Autodesk Inventor part; units mm, degrees
ref_plane "YZ Plane" through (0, 0, 0) normal (1, 0, 0) x (0, 1, 0)
ref_plane "XZ Plane" through (0, 0, 0) normal (0, 1, 0) x (-1, 0, 0)
ref_plane "XY Plane" through (0, 0, 0) normal (0, 0, 1) x (1, 0, 0)
sketch "Sketch1" plane through (0, 0, 0) normal (0, 0, 1) x (1, 0, 0)
  line L0 (0, 0) -> (419.7625, 0)
  line L1 (419.7625, 0) -> (419.7625, 420)
  line L2 (419.7625, 420) -> (0, 420)
  line L3 (0, 420) -> (0, 0)
  dimension "d0" = 419.7625
  dimension "d1" = 420
extrude "Extrusion1" add sketch "Sketch1" along normal blind 4.7625
sketch "Sketch3" plane through (0, 0, 4.7625) normal (0, 0, 1) x (1, 0, 0)
  line L0 (0, 0) -> (419.7625, 0)
  line L1 (0, 420) -> (0, 0)
  circle A0 centre (209.8815, 40) radius 19.05
  dimension "d13" = 38.1
  dimension "d14" = 209.8815
  dimension "d30" = 40
extrude "Extrusion2" cut sketch "Sketch3" against normal up to next
sketch "Sketch5" plane through (0, 0, 4.7625) normal (0, 0, 1) x (1, 0, 0)
  circle A0 centre (209.8815, 40) radius 19.05
  point P0 (193.8815, 56)
  point P1 (225.8815, 56)
  point P2 (193.8815, 24)
  point P3 (225.8815, 24)
  dimension "d31" = 32
  dimension "d32" = 32
  dimension "d33" = 16
  dimension "d34" = 16
hole "Hole2" at (193.8815, 56, 4.7625) at (225.8815, 56, 4.7625) at (193.8815, 24, 4.7625) at (225.8815, 24, 4.7625) direction (0, 0, -1) diameter 3.5 end through all
sketch "Sketch6" plane through (0, 0, 4.7625) normal (0, 0, 1) x (1, 0, 0)
  line L0 (0, 0) -> (419.7625, 0)
  line L1 (419.7625, 0) -> (419.7625, 420)
  line L2 (419.7625, 420) -> (0, 420)
  line L3 (0, 420) -> (0, 0)
  circle A0 centre (10, 410) radius 2.25
  circle A1 centre (409.7625, 410) radius 2.25
  circle A2 centre (10, 10) radius 2.25
  circle A3 centre (409.7625, 10) radius 2.25
  circle A4 centre (10, 210) radius 2.25
  circle A5 centre (409.7625, 210) radius 2.25
  circle A6 centre (209.8815, 410) radius 2.25
  circle A7 centre (209.8815, 10) radius 2.25
  circle A8 centre (209.8815, 75) radius 2.25
  dimension "d42" = 4.5
  dimension "d43" = 10
  dimension "d44" = 10
  dimension "d45" = 10
  dimension "d46" = 10
  dimension "d47" = 10
  dimension "d48" = 210
  dimension "d51" = 209.8815
  dimension "d55" = 75
extrude "Extrusion3" cut sketch "Sketch6" against normal up to next contours A0 | A1 | A2 | A3 | A4 | A5 | A6 | A7 | A8
chamfer "Chamfer1" distance 2 angle 45 9 edges at (7.75, 410, 4.7625) (207.6315, 410, 4.7625) (407.5125, 410, 4.7625) (407.5125, 210, 4.7625) (7.75, 210, 4.7625) (7.75, 10, 4.7625) (207.6315, 10, 4.7625) (407.5125, 10, 4.7625) (207.6315, 75, 4.7625)
properties part number "EnclosurePanelSide" material "ABS Plastic"
Work out the finished part from the listing and answer in its coordinate system (mm). Coordinates: 2 decimals unless noted, no trailing zeros. Use a Markdown table: item, result.
Item 1: Given pin 1 Ø2 at (x, y) = (225.88, 24) entering from +Z; pin 2 Ø6 at (x, y) = (409.76, 10) entering from +Z (3 decimals); pin 3 Ø5 at (x, y) = (10, 410) entering from +Z; pin 4 Ø7 at (x, y) = (10, 10) entering from +Z, each flat-ended and moving along its own axis, determine where each tip first touches the part or whether it passes through.
Evaluation:
| item | result |
|---|---|
| pin 1 | passes through |
| pin 2 | stops at z = 3.515 |
| pin 3 | stops at z = 3.01 |
| pin 4 | stops at z = 4.01 |
Item 2: The mould has two halves that part along Y. Classify faces 1 (the flat face through (207, 213, 0)), 2 (the cylindrical face through (228.052, 45.722, 2.415)): +Y half, -Y half, draft (parallel to the pull), parting line (faces both ways), or undercut.
Evaluation:
| item | result |
|---|---|
| face 1 | draft |
| face 2 | undercut |
Item 3: Consider probe 1 along X at (y, z) = (410, 1.6); probe 2 along X at (y, z) = (210, 0.7); probe 3 along Y at (x, z) = (221, 0.25). Determine where each line is inside the solid, lowest interval first. Write a range as from..to.
Evaluation:
| item | result |
|---|---|
| probe 1 | x = 0..7.75, 12.25..207.63, 212.13..407.51, 412.01..419.76 |
| probe 2 | x = 0..7.75, 12.25..407.51, 412.01..419.76 |
| probe 3 | y = 0..24.53, 55.47..420 |
